```python
from build123d import *

# Parameters (mm, degrees)
SKETCH_1_W          = 20
SKETCH_1_H          = 20
SKETCH_1_W_2        = 18
SKETCH_1_H_2        = 18
EXTRUDE_1_DEPTH     = 1360
SKETCH_2_R          = 1.6
CUT_EXTRUDE_1_DEPTH = 1361.294085851
SKETCH_3_R          = 1.6
CUT_EXTRUDE_2_DEPTH = 1361.294085851


with BuildPart() as part:
    # 草图1 → 凸台-拉伸1 (new body)
    with BuildSketch(Plane.XY):
        with Locations((10, 10)):
            Rectangle(SKETCH_1_W, SKETCH_1_H)
        with Locations((10, 10)):
            Rectangle(SKETCH_1_W_2, SKETCH_1_H_2, mode=Mode.SUBTRACT)
    extrude(amount=EXTRUDE_1_DEPTH)

    # 草图2 → 切除-拉伸1 (cut, through all)
    with BuildSketch(Plane(origin=(0, 20, 0), x_dir=(1, 0, 0), z_dir=(0, 1, 0))):
        with Locations(Location((11, -15.5, 0), (0, 0, 270))):
            Circle(SKETCH_2_R)
        with Locations(Location((11, -8.5, 0), (0, 0, 270))):
            Circle(SKETCH_2_R)
        with Locations(Location((11, -71.5, 0), (0, 0, 270))):
            Circle(SKETCH_2_R)
        with Locations(Location((11, -64.5, 0), (0, 0, 270))):
            Circle(SKETCH_2_R)
        with Locations(Location((11, -1295.5, 0), (0, 0, 270))):
            Circle(SKETCH_2_R)
        with Locations(Location((11, -1288.5, 0), (0, 0, 270))):
            Circle(SKETCH_2_R)
        with Locations(Location((11, -1351.5, 0), (0, 0, 270))):
            Circle(SKETCH_2_R)
        with Locations(Location((11, -1344.5, 0), (0, 0, 270))):
            Circle(SKETCH_2_R)
    extrude(amount=-CUT_EXTRUDE_1_DEPTH, mode=Mode.SUBTRACT)

    # 草图3 → 切除-拉伸2 (cut, through all)
    with BuildSketch(Plane.XZ):
        with Locations(Location((12, 1312, 0), (0, 0, 270))):
            Circle(SKETCH_3_R)
        with Locations(Location((12, 1328, 0), (0, 0, 270))):
            Circle(SKETCH_3_R)
        with Locations(Location((12, 32, 0), (0, 0, 270))):
            Circle(SKETCH_3_R)
        with Locations(Location((12, 48, 0), (0, 0, 270))):
            Circle(SKETCH_3_R)
        with Locations(Location((5, 1312, 0), (0, 0, 270))):
            Circle(SKETCH_3_R)
        with Locations(Location((5, 1328, 0), (0, 0, 270))):
            Circle(SKETCH_3_R)
        with Locations(Location((5, 32, 0), (0, 0, 270))):
            Circle(SKETCH_3_R)
        with Locations(Location((5, 48, 0), (0, 0, 270))):
            Circle(SKETCH_3_R)
    extrude(amount=-CUT_EXTRUDE_2_DEPTH, mode=Mode.SUBTRACT)


solid = part.part
```
For this review, take the finished solid that the model builds, in its own axes (mm). Coordinates: 2 decimals unless noted, no trailing zeros. Loops run counter-clockwise (first coordinate to the right, second up) from the corner with the lowest first, then second, coordinate; pieces in that order, holes last. Notation, with made-up numbers: (10, 49) - (67, 49) arc R15 ccw to (67, 69) - close; hole circle Ø4 at (2.5, 6.25). An arc over 180 degrees is marked (long way). Use one line per item in the form item = value. Start each with the question number.
1) To check wall thickness, follow probe 1 along X at (y, z) = (0.25, 48); probe 2 along Y at (x, z) = (2.75, 1053.5). State the ranges of each line that lie inside material, in increasing order. Write a range as from..to.
2) Take a section at B-B (z = 746). State the section outline as (x, y) points, plus the area to 3 significant figures.
3) For pin 1 (5 mm diameter, centred on x = 11, z = 15.5, fed in from -Y), flat-tipped, find the tip position at first contact; note if it passes through.
4) Take a section at A-A (y = 9.5). State the section outline as (x, z) points.
From the geometry:
q1.probe_1 = 0..3.4, 6.6..10.4, 13.6..20
q1.probe_2 = 0..1, 19..20
q2.outline = (0, 0) - (20, 0) - (20, 20) - (0, 20) - close; hole (1, 1) - (19, 1) - (19, 19) - (1, 19) - close
q2.area = 76.0 mm2
q3.pin_1 = 0
q4.outline = (0, 0) - (1, 0) - (1, 1360) - (0, 1360) - close; (19, 0) - (20, 0) - (20, 1360) - (19, 1360) - close
